Geometry check sheet. Reference: the model listing, model coordinates, mm. A direction names the side the tool comes from. Round coordinates to 2 decimals unless told otherwise and drop trailing zeros. Write each loop counter-clockwise with the first axis right and the second up, starting at its lowest first coordinate (ties: lowest second). Pieces come first, ordered by that corner, then holes. Notation, with made-up numbers: (17, -26.5) -> (23, -26.5) arc R22 cw to (23, -5.5) -> close; hole circle Ø5 at (87, -25). An arc over 180 degrees is marked (long way). Use a Markdown table: item, result.
```python
from build123d import *

# Parameters (mm, degrees)
SKETCH1_W           = 3.175
SKETCH1_H           = 25.4
SKETCH1_W_2         = 28.575
SKETCH1_H_2         = 3.175
BOSS_EXTRUDE1_DEPTH = 50.8
POT_MOUNT_REACH     = 5.175
SKETCH2_R           = 3.683
BASE_MOUNT_REACH    = 5.175
SKETCH3_R           = 3.96875


with BuildPart() as part:
    # Sketch1 → Boss-Extrude1 (new body)
    with BuildSketch(Plane.XY):
        with Locations((1.5875, 12.7)):
            Rectangle(SKETCH1_W, SKETCH1_H)
        with Locations((17.4625, 1.5875)):
            Rectangle(SKETCH1_W_2, SKETCH1_H_2)
    extrude(amount=BOSS_EXTRUDE1_DEPTH)

    # Sketch2 → Pot Mount (cut, up to next)
    with BuildSketch(Plane(origin=(3.175, 0, 0), x_dir=(0, 0, -1), z_dir=(1, 0, 0)), mode=Mode.PRIVATE) as pot_mount_sk1:
        with Locations((-25.4, 13.97)):
            Circle(SKETCH2_R)
    pot_mount_tool1 = extrude(pot_mount_sk1.sketch, amount=-POT_MOUNT_REACH, mode=Mode.PRIVATE) & part.part
    add(pot_mount_tool1.solids().sort_by_distance((3.175, 13.97, 25.4))[0], mode=Mode.SUBTRACT)

    # Sketch3 → Base Mount (cut, up to next)
    with BuildSketch(Plane(origin=(0, 3.175, 0), x_dir=(1, 0, 0), z_dir=(0, 1, 0)), mode=Mode.PRIVATE) as base_mount_sk1:
        with Locations((22.225, -38.1)):
            Circle(SKETCH3_R)
    base_mount_tool1 = extrude(base_mount_sk1.sketch, amount=-BASE_MOUNT_REACH, mode=Mode.PRIVATE) & part.part
    add(base_mount_tool1.solids().sort_by_distance((22.225, 3.175, 38.1))[0], mode=Mode.SUBTRACT)
    # Sketch3 → Base Mount (cut, up to next)
    with BuildSketch(Plane(origin=(0, 3.175, 0), x_dir=(1, 0, 0), z_dir=(0, 1, 0)), mode=Mode.PRIVATE) as base_mount_sk2:
        with Locations((22.225, -12.7)):
            Circle(SKETCH3_R)
    base_mount_tool2 = extrude(base_mount_sk2.sketch, amount=-BASE_MOUNT_REACH, mode=Mode.PRIVATE) & part.part
    add(base_mount_tool2.solids().sort_by_distance((22.225, 3.175, 12.7))[0], mode=Mode.SUBTRACT)


solid = part.part
```
(1) Section check D-D on y = 19.75. Record the cut outline in (x, z) (3 decimals).
A:
| item | result |
|---|---|
| outline | (0, 0) -> (3.175, 0) -> (3.175, 50.8) -> (0, 50.8) -> close |
(2) Section check B-B on z = 12.7. Record the cut outline in (x, y) (3 decimals).
A:
| item | result |
|---|---|
| outline | (0, 0) -> (18.256, 0) -> (18.256, 3.175) -> (3.175, 3.175) -> (3.175, 25.4) -> (0, 25.4) -> close; (26.194, 0) -> (31.75, 0) -> (31.75, 3.175) -> (26.194, 3.175) -> close |
(3) Section check C-C on z = 25.4. Record the cut outline in (x, y) (3 decimals).
A:
| item | result |
|---|---|
| outline | (0, 0) -> (31.75, 0) -> (31.75, 3.175) -> (3.175, 3.175) -> (3.175, 10.287) -> (0, 10.287) -> close; (0, 17.653) -> (3.175, 17.653) -> (3.175, 25.4) -> (0, 25.4) -> close |
(4) Access from +Z, -Z, +X, -X, +Y, -Y to the whole of each face (thin tool, end or side, straight path). Record for faces 4 (the face through (3.175, 19, 25)), 5 (the face through (18.26, 1.61, 12.53)).
A:
| item | result |
|---|---|
| face 4 | +Z, -Z, +X, +Y |
| face 5 | +Y, -Y |
(5) Section check A-A on y = 13.97. Record the cut outline in (x, z) (3 decimals).
A:
| item | result |
|---|---|
| outline | (0, 0) -> (3.175, 0) -> (3.175, 21.717) -> (0, 21.717) -> close; (0, 29.083) -> (3.175, 29.083) -> (3.175, 50.8) -> (0, 50.8) -> close |
(6) Release check for a two-part mould opening along X. For faces 1 (the face through (19.076, 1.61, 40.515)), 2 (the face through (16, 0, 25)), 3 (the face through (31.75, 2, 25)) record: +X half, -X half, draft (parallel to the pull), parting line (faces both ways), or undercut.
A:
| item | result |
|---|---|
| face 1 | undercut |
| face 2 | draft |
| face 3 | +X half |
(7) Thickness scan on line 1 (X direction, y = 1.3, z = 12.7); line 2 (X direction, y = 12.75, z = 33.5) (3 decimals); line 3 (Z direction, x = 2, y = 13.5). Record the ranges inside material, lowest first.
A:
| item | result |
|---|---|
| line 1 | x = 0 to 18.26, 26.19 to 31.75 |
| line 2 | x = 0 to 3.175 |
| line 3 | z = 0 to 21.75, 29.05 to 50.8 |
(8) Gauge pin test, flat ends, axial feed: pin 1 Ø2 at (x, z) = (27.5, 29.5) entering from +Y (3 decimals); pin 2 Ø12 at (y, z) = (13.97, 25.4) entering from +X (3 decimals). Record the tip position at first contact, or that the pin passes through.
A:
| item | result |
|---|---|
| pin 1 | stops at y = 3.175 |
| pin 2 | stops at x = 3.175 |
